from build123d import *

# Parameters (mm, degrees)
F1_DEPTH       = 63.5
F0_W           = 24.1773966307
F0_H           = 19.05
F2_DEPTH       = 25.4
F3_DEPTH       = 7.9375
F5_R           = 6.35
F7_D           = 6.7564
F7_CSINK_D     = 13.4874
F7_CSINK_ANGLE = 82


with BuildPart() as f1:
    # F0 (on Front) → F1 (new body, symmetric)
    with BuildSketch(Plane.XZ):
        Polygon((22.225, 9.525), (-41.275, 9.525), (-41.275, -9.525), (41.275, -9.525), (41.275, 9.525), align=None)
    extrude(amount=F1_DEPTH, both=True)

    # F0 (on Front) → F2 (join, symmetric)
    with BuildSketch(Plane.XZ):
        with BuildLine():
            Line((22.225, 27.0002), (22.225, 9.525))
            Line((22.225, 9.525), (41.275, 9.525))
            Line((41.275, 9.525), (41.275, 27.0002))
            ThreePointArc((41.275, 27.0002), (45.9246798487, 38.2255201513), (57.15, 42.8752))
            Line((57.15, 42.8752), (60.325, 42.8752))
            Line((60.325, 42.8752), (60.325, 61.9252))
            Line((60.325, 61.9252), (57.15, 61.9252))
            add(Edge.make_bspline(
                [(56.1585534781, 61.9111246339), (56.4889663623, 61.9166719821), (56.8194531057, 61.9213645655), (57.15, 61.9252)],
                knots=[110.7679621102, 110.7679621102, 110.7679621102, 110.7679621102, 111.5045361635, 111.5045361635, 111.5045361635, 111.5045361635], degree=3))
            ThreePointArc((56.1585534781, 61.9111246339), (32.1062193871, 51.3428514088), (22.225, 27.0002))
        make_face()
        with Locations((72.4136983154, 52.4002)):
            Rectangle(F0_W, F0_H)
    extrude(amount=F2_DEPTH, both=True)

    # F0 (on Front) → F3 (join, symmetric)
    with BuildSketch(Plane.XZ):
        with BuildLine():
            add(Edge.make_bspline(
                [(-41.275, 9.525), (-41.5478571248, 40.9122167506), (6.4701865541, 61.0768996786), (56.1585534781, 61.9111246339)],
                knots=[0, 0, 0, 0, 110.7679621102, 110.7679621102, 110.7679621102, 110.7679621102], degree=3))
            Line((-41.275, 9.525), (22.225, 9.525))
            Line((22.225, 9.525), (22.225, 27.0002))
            ThreePointArc((22.225, 27.0002), (32.1062193871, 51.3428514088), (56.1585534781, 61.9111246339))
        make_face()
    extrude(amount=F3_DEPTH, both=True)

    # F0 (on Front) → F4 (revolve)
    with BuildSketch(Plane.XZ):
        Polygon((84.5023966307, 66.675), (84.5023966307, 61.9252), (84.5023966307, 42.8752), (84.5023966307, 38.1), (111.125, 38.1), (111.125, 66.675), align=None)
    revolve(axis=Axis((84.5023966307, 0, 52.3875), (0, 0, 1)))

    # F5
    f5_edges = [f1.edges().sort_by_distance(p)[0] for p in [
        (-41.275, -63.5, 0),
        (41.275, -63.5, 0),
        (-41.275, 63.5, 0),
        (41.275, 63.5, 0),
    ]]
    fillet(f5_edges, radius=F5_R)

    # F7 (through all)
    with Locations(Plane.XY.offset(9.525)):
        with Locations((-28.575, 50.8), (28.575, 50.8), (-28.575, -50.8), (28.575, -50.8)):
            CounterSinkHole(F7_D / 2, F7_CSINK_D / 2, counter_sink_angle=F7_CSINK_ANGLE)


solid = f1.part
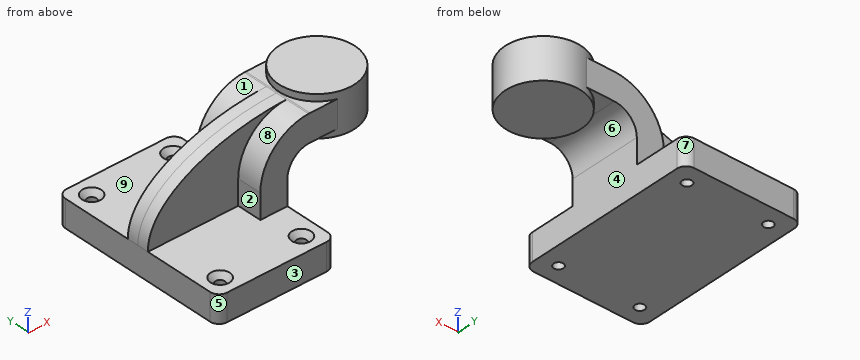
Read the model definition and answer for the solid it produces. Units are mm, in the model's axes. Face numbers are marked on the shaded views. A direction names the side the tool comes from. Round coordinates to 2 decimals unless told otherwise and drop trailing zeros. Order: outer loops, then holes, each group sorted by start corner. A loop starts at its lowest first (then second) coordinate and runs counter-clockwise, first axis right, second up.
1) The mould has two halves that part along X. Classify the marked faces 6, 7, 8 and 9: released by +X, released by -X, zero draft, split by the parting line, or undercut.
2) Flat-ended cylindrical pins translate along their axes: pin 1 (2 mm diameter, centred on x = -1, z = 49, fed in from +Y); pin 2 (5 mm diameter, centred on y = 18.5, z = 16.5, fed in from -X) (3 decimals); pin 3 (5 mm diameter, centred on x = 83.5, z = 39.5, fed in from -Y); pin 4 (5.5 mm diameter, centred on x = -28.575, y = -50.8, fed in from -Z) (3 decimals). Find the tip coordinate at first contact, or state that the pin passes through.
3) For the marked faces 1, 2, 3, 4 and 5, determine the directions among +Z, -Z, +X, -X, +Y, -Y from which every point of the face is accessible in a straight line to the end or side of a thin tool.
4) The part is cut by section A-A on y = -50.8. Write down the section's boundary in (x, z) (3 decimals).
5) The part is cut by section B-B on x = 85.5. Write down the section's boundary in (y, z) (3 decimals).
6) Straight lines are drawn through the part: L1, parallel to X at y = 50.8, z = -1 (3 decimals); L2, parallel to X at y = -50, z = 0 (3 decimals); L3, parallel to Z at x = 69, y = -21 (3 decimals). For each, find the intervals that lie inside material, in ascending order.
Resolved:
1. face 6: undercut
1. face 7: released by +X
1. face 8: released by -X
1. face 9: zero draft
2. pin 1: stops at y = 7.94
2. pin 2: stops at x = 22.225
2. pin 3: stops at y = -26.62
2. pin 4: passes through
3. face 1: +Z, -X, +Y
3. face 2: +Z, -X, -Y
3. face 3: +Z, -Z, +X, -X, -Y
3. face 4: -Z, +X, +Y, -Y
3. face 5: +Z, -Z, -X, -Y
4. outline: (-41.275, -9.525) - (-31.953, -9.525) - (-31.953, 5.653) - (-35.319, 9.525) - (-41.275, 9.525) - close; (-25.197, -9.525) - (25.197, -9.525) - (25.197, 5.653) - (21.831, 9.525) - (-21.831, 9.525) - (-25.197, 5.653) - close; (31.953, -9.525) - (41.275, -9.525) - (41.275, 9.525) - (35.319, 9.525) - (31.953, 5.653) - close
5. outline: (-26.604, 38.1) - (26.604, 38.1) - (26.604, 66.675) - (-26.604, 66.675) - close
6. L1: x = -41.275 to -31.953, -25.197 to 25.197, 31.953 to 41.275
6. L2: x = -41.275 to -31.857, -25.293 to 25.293, 31.857 to 41.275
6. L3: z = 38.1 to 66.675
